Check sheet for the modelled part. Datum: model origin and axes. Units: mm. Face numbers are marked on the shaded views. A direction names the side the tool comes from. Round coordinates to 2 decimals unless told otherwise and drop trailing zeros. Loops run counter-clockwise (first coordinate to the right, second up) from the corner with the lowest first, then second, coordinate; pieces in that order, holes last. Notation, with made-up numbers: (-28.5, 70) -> (-8.5, 70) arc R33 ccw to (-8.5, 102) -> close; hole circle Ø3 at (50.25, 4.5). An arc over 180 degrees is marked (long way). One line per question, with ' | ' between items.
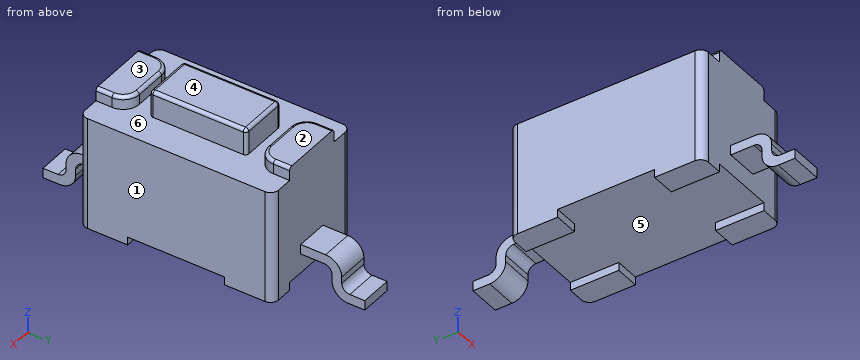
```python
from build123d import *

# Parameters (mm, degrees)
SKETCH1_W            = 3.5
SKETCH1_H            = 6
BOSS_EXTRUDE1_DEPTH  = 3.25
SKETCH2_W            = 1
SKETCH2_H            = 0.3
BOSS_EXTRUDE2_DEPTH  = 1.9845
SKETCH3_W            = 1
SKETCH3_H            = 1.0145
BOSS_EXTRUDE3_DEPTH  = 0.95
SKETCH4_W            = 1
SKETCH4_H            = 0.3
BOSS_EXTRUDE4_DEPTH  = 1.9845
SKETCH5_W            = 1
SKETCH5_H            = 1.0145
BOSS_EXTRUDE5_DEPTH  = 0.95
SKETCH6_W            = 0.95
SKETCH6_H            = 0.7145
CUT_EXTRUDE1_DEPTH   = 8.028510884
SKETCH7_W            = 0.95
SKETCH7_H            = 0.7145
CUT_EXTRUDE2_DEPTH   = 8.028510884
SKETCH8_W            = 0.75
SKETCH8_H            = 1.5
BOSS_EXTRUDE6_DEPTH  = 0.25
SKETCH9_W            = 0.75
SKETCH9_H            = 1.5
BOSS_EXTRUDE7_DEPTH  = 0.25
SKETCH10_W           = 0.75
SKETCH10_H           = 1.5
BOSS_EXTRUDE8_DEPTH  = 0.25
SKETCH11_W           = 0.75
SKETCH11_H           = 1.5
BOSS_EXTRUDE9_DEPTH  = 0.25
SKETCH12_W           = 2
SKETCH12_H           = 1
BOSS_EXTRUDE10_DEPTH = 0.4075
SKETCH13_W           = 2
SKETCH13_H           = 1
BOSS_EXTRUDE11_DEPTH = 0.4075
SKETCH14_W           = 1.52
SKETCH14_H           = 3
BOSS_EXTRUDE12_DEPTH = 0.815
FILLET1_R            = 0.5
FILLET2_R            = 0.1
FILLET3_R            = 0.25


with BuildPart() as part:
    # Sketch1 → Boss-Extrude1 (new body)
    with BuildSketch(Plane(origin=(0, 0, -4.065), x_dir=(-1, 0, 0), z_dir=(0, 0, -1))):
        Rectangle(SKETCH1_W, SKETCH1_H)
    extrude(amount=-BOSS_EXTRUDE1_DEPTH)

    # Sketch2 → Boss-Extrude2 (add)
    with BuildSketch(Plane(origin=(0, 3, 0), x_dir=(-1, 0, 0), z_dir=(0, 1, 0))):
        with Locations((0, -3.315)):
            Rectangle(SKETCH2_W, SKETCH2_H)
    extrude(amount=BOSS_EXTRUDE2_DEPTH)

    # Sketch3 → Boss-Extrude3 (add)
    with BuildSketch(Plane(origin=(0, 0, -3.465), x_dir=(-1, 0, 0), z_dir=(0, 0, -1))):
        with Locations((0, 4.47725)):
            Rectangle(SKETCH3_W, SKETCH3_H)
    extrude(amount=BOSS_EXTRUDE3_DEPTH)

    # Sketch4 → Boss-Extrude4 (add)
    with BuildSketch(Plane.XZ.offset(3)):
        with Locations((0, -3.315)):
            Rectangle(SKETCH4_W, SKETCH4_H)
    extrude(amount=BOSS_EXTRUDE4_DEPTH)

    # Sketch5 → Boss-Extrude5 (add)
    with BuildSketch(Plane(origin=(0, 0, -3.465), x_dir=(-1, 0, 0), z_dir=(0, 0, -1))):
        with Locations((0, -4.47725)):
            Rectangle(SKETCH5_W, SKETCH5_H)
    extrude(amount=BOSS_EXTRUDE5_DEPTH)

    # Sketch6 → Cut-Extrude1 (cut, through all)
    with BuildSketch(Plane(origin=(0.5, 0, 0), x_dir=(0, 0, -1), z_dir=(1, 0, 0))):
        with Locations((3.64, 4.62725)):
            Rectangle(SKETCH6_W, SKETCH6_H)
    extrude(amount=-CUT_EXTRUDE1_DEPTH, mode=Mode.SUBTRACT)

    # Sketch7 → Cut-Extrude2 (cut, through all)
    with BuildSketch(Plane(origin=(0.5, 0, 0), x_dir=(0, 0, -1), z_dir=(1, 0, 0))):
        with Locations((3.64, -4.62725)):
            Rectangle(SKETCH7_W, SKETCH7_H)
    extrude(amount=-CUT_EXTRUDE2_DEPTH, mode=Mode.SUBTRACT)

    # Sketch8 → Boss-Extrude6 (add)
    with BuildSketch(Plane(origin=(0, 0, -4.065), x_dir=(-1, 0, 0), z_dir=(0, 0, -1))):
        with Locations((-1.375, 2.25)):
            Rectangle(SKETCH8_W, SKETCH8_H)
    extrude(amount=BOSS_EXTRUDE6_DEPTH)

    # Sketch9 → Boss-Extrude7 (add)
    with BuildSketch(Plane(origin=(0, 0, -4.065), x_dir=(-1, 0, 0), z_dir=(0, 0, -1))):
        with Locations((-1.375, -2.25)):
            Rectangle(SKETCH9_W, SKETCH9_H)
    extrude(amount=BOSS_EXTRUDE7_DEPTH)

    # Sketch10 → Boss-Extrude8 (add)
    with BuildSketch(Plane(origin=(0, 0, -4.065), x_dir=(-1, 0, 0), z_dir=(0, 0, -1))):
        with Locations((1.375, 2.25)):
            Rectangle(SKETCH10_W, SKETCH10_H)
    extrude(amount=BOSS_EXTRUDE8_DEPTH)

    # Sketch11 → Boss-Extrude9 (add)
    with BuildSketch(Plane(origin=(0, 0, -4.065), x_dir=(-1, 0, 0), z_dir=(0, 0, -1))):
        with Locations((1.375, -2.25)):
            Rectangle(SKETCH11_W, SKETCH11_H)
    extrude(amount=BOSS_EXTRUDE9_DEPTH)

    # Sketch12 → Boss-Extrude10 (add)
    with BuildSketch(Plane.XY.offset(-0.815)):
        with Locations((0, -2.5)):
            Rectangle(SKETCH12_W, SKETCH12_H)
    extrude(amount=BOSS_EXTRUDE10_DEPTH)

    # Sketch13 → Boss-Extrude11 (add)
    with BuildSketch(Plane.XY.offset(-0.815)):
        with Locations((0, 2.5)):
            Rectangle(SKETCH13_W, SKETCH13_H)
    extrude(amount=BOSS_EXTRUDE11_DEPTH)

    # Sketch14 → Boss-Extrude12 (add)
    with BuildSketch(Plane.XY.offset(-0.815)):
        Rectangle(SKETCH14_W, SKETCH14_H)
    extrude(amount=BOSS_EXTRUDE12_DEPTH)

    # Fillet1
    fillet1_edges = [part.edges().sort_by_distance(p)[0] for p in [
        (0, 3.97, -4.415),
        (0, 4.27, -3.165),
        (0, -4.27, -3.165),
        (0, -3.97, -4.415),
        (-1, 2, -0.61125),
        (1, -2, -0.61125),
        (-1, -2, -0.61125),
        (1, 2, -0.61125),
    ]]
    fillet(fillet1_edges, radius=FILLET1_R)

    # Fillet2
    fillet2_edges = [part.edges().sort_by_distance(p)[0] for p in [
        (-0.76, -1.5, -0.4075),
        (0.76, -1.5, -0.4075),
        (0, -1.5, 0),
        (-0.76, 0, 0),
        (-0.76, 1.5, -0.4075),
        (0.76, 0, 0),
        (0, 1.5, 0),
        (0.76, 1.5, -0.4075),
        (-1, 2.75, -0.4075),
        (-0.853553391, 2.146446609, -0.4075),
        (0, 2, -0.4075),
        (0.853553391, 2.146446609, -0.4075),
        (1, 2.75, -0.4075),
        (1, -2.75, -0.4075),
        (0.853553391, -2.146446609, -0.4075),
        (0, -2, -0.4075),
        (-1, -2.75, -0.4075),
        (-0.853553391, -2.146446609, -0.4075),
    ]]
    fillet(fillet2_edges, radius=FILLET2_R)

    # Fillet3
    fillet3_edges = [part.edges().sort_by_distance(p)[0] for p in [
        (0, -4.27, -4.115),
        (-1.75, -3, -2.565),
        (-1.75, 3, -2.565),
        (1.75, -3, -2.565),
        (1.75, 3, -2.565),
        (0, 4.27, -4.115),
        (0, -3.97, -3.465),
        (0, 3.97, -3.465),
    ]]
    fillet(fillet3_edges, radius=FILLET3_R)


solid = part.part
```
(1) Scan lines: probe 1 along Y at (x, z) = (-0.3, -0.65); probe 2 along Y at (x, z) = (0.25, -4); probe 3 along Y at (x, z) = (-0.6, -0.2). Record each from-to range of solid material in increasing order.
Answer:
probe 1: y = -3 to -2, -1.5 to 1.5, 2 to 3 | probe 2: y = -4.31 to -3.98, -3 to 3, 3.98 to 4.31 | probe 3: y = -1.5 to 1.5
(2) Sectioned sample at C-C, the plane z = -2.1. Record the cut outline in (x, y), and give its area (3 significant figures).
Answer:
outline: (-1.75, -2.75) arc R0.25 ccw to (-1.5, -3) -> (1.5, -3) arc R0.25 ccw to (1.75, -2.75) -> (1.75, 2.75) arc R0.25 ccw to (1.5, 3) -> (-1.5, 3) arc R0.25 ccw to (-1.75, 2.75) -> close | area: 20.9 mm2
(3) Set-up check for the marked faces 1, 2 and 3: record each of +Z, -Z, +X, -X, +Y, -Y from which the full face is reachable in a straight line by a thin tool's end or side.
Answer:
face 1: +Z, -Z, +X, +Y, -Y | face 2: +Z, +X, -X, +Y | face 3: +Z, +X, -X, -Y
(4) Sectioned sample at D-D, the plane z = -3.3. Record the cut outline in (x, y).
Answer:
outline: (-1.75, -2.75) arc R0.25 ccw to (-1.5, -3) -> (-0.5, -3) -> (-0.5, -4.11) -> (0.5, -4.11) -> (0.5, -3) -> (1.5, -3) arc R0.25 ccw to (1.75, -2.75) -> (1.75, 2.75) arc R0.25 ccw to (1.5, 3) -> (0.5, 3) -> (0.5, 4.11) -> (-0.5, 4.11) -> (-0.5, 3) -> (-1.5, 3) arc R0.25 ccw to (-1.75, 2.75) -> close
(5) Sectioned sample at A-A, the plane y = -1. Record the cut outline in (x, z) (3 decimals), and give its area (3 significant figures).
Answer:
outline: (-1.75, -4.065) -> (1.75, -4.065) -> (1.75, -0.815) -> (0.76, -0.815) -> (0.76, -0.1) arc R0.1 ccw to (0.66, 0) -> (-0.66, 0) arc R0.1 ccw to (-0.76, -0.1) -> (-0.76, -0.815) -> (-1.75, -0.815) -> close | area: 12.6 mm2
(6) Mould release check, pull along Y, two halves, no side actions. Record for the marked faces 4, 5 and 6: +Y half, -Y half, draft (parallel to the pull), parting line (faces both ways), or undercut.
Answer:
face 4: draft | face 5: undercut | face 6: undercut
(7) Go/stop test with flat-tipped pins: pin 1 (0.6 mm diameter, centred on x = 0, y = -3.5, fed in from +Z) (3 decimals); pin 2 (0.9 mm diameter, centred on x = 0.5, z = -2.5, fed in from +Y); pin 3 (0.8 mm diameter, centred on x = -1, y = 2, fed in from -Z) (3 decimals). Record where each tip stops, or that it passes through.
Answer:
pin 1: stops at z = -3.165 | pin 2: stops at y = 3 | pin 3: stops at z = -4.315
(8) Sectioned sample at B-B, the plane x = -1.2. Record the cut outline in (y, z) (3 decimals).
Answer:
outline: (-3, -4.315) -> (-1.5, -4.315) -> (-1.5, -4.065) -> (1.5, -4.065) -> (1.5, -4.315) -> (3, -4.315) -> (3, -0.815) -> (-3, -0.815) -> close
